from build123d import *
from OCP.BRepFilletAPI import BRepFilletAPI_MakeChamfer

# Parameters (mm, degrees)
SKETCH2_R           = 31
SKETCH2_R_2         = 25
SKETCH2_R_3         = 4
SKETCH2_R_4         = 3
SKETCH2_R_5         = 3.333333333
BOSS_EXTRUDE1_DEPTH = 10
BOSS_EXTRUDE2_START = 50
SKETCH2_3_R         = 31
SKETCH2_3_R_2       = 25
BOSS_EXTRUDE2_DEPTH = 50
FILLET1_R           = 6
SKETCH3_R           = 7
CUT_EXTRUDE1_DEPTH  = 3
BOSS_EXTRUDE3_DEPTH = 6
CIRPATTERN1_COUNT   = 6
BOSS_EXTRUDE4_START = 44
SKETCH6_R           = 70
SKETCH6_R_2         = 55
BOSS_EXTRUDE4_DEPTH = 6
CHAMFER1_SIZE       = 12.228610788
CHAMFER1_SIZE_2     = 24
CUT_EXTRUDE2_DEPTH  = 6
CIRPATTERN2_COUNT   = 12


with BuildPart() as part:
    # Sketch2 → Boss-Extrude1 (new body)
    # profile 1 of 2: a face of its own
    with BuildSketch(Plane(origin=(0, 0, 0), x_dir=(1, 0, 0), z_dir=(0, 1, 0))):
        with Locations(Location((0, 0, 0), (0, 0, 270))):
            Circle(SKETCH2_R)
        Circle(SKETCH2_R_2, mode=Mode.SUBTRACT)
    # profile 2 of 2: a face of its own
    with BuildSketch(Plane(origin=(0, 0, 0), x_dir=(1, 0, 0), z_dir=(0, 1, 0))):
        Circle(SKETCH2_R_2)
        with Locations(Location((0, 0, 0), (0, 0, 270))):
            Circle(SKETCH2_R_3, mode=Mode.SUBTRACT)
        with Locations(Location((-16, 0, 0), (0, 0, 270))):
            Circle(SKETCH2_R_4, mode=Mode.SUBTRACT)
        with Locations(Location((16, 0, 0), (0, 0, 270))):
            Circle(SKETCH2_R_5, mode=Mode.SUBTRACT)
    extrude(amount=-BOSS_EXTRUDE1_DEPTH)

    # Sketch2<3> → Boss-Extrude2 (add)
    with BuildSketch(Plane(origin=(0, 0, 0), x_dir=(1, 0, 0), z_dir=(0, 1, 0)).offset(BOSS_EXTRUDE2_START)):
        with Locations(Location((0, 0, 0), (0, 0, 270))):
            Circle(SKETCH2_3_R)
        with Locations(Location((0, 0, 0), (0, 0, 270))):
            Circle(SKETCH2_3_R_2, mode=Mode.SUBTRACT)
    extrude(amount=-BOSS_EXTRUDE2_DEPTH)

    # Fillet1
    fillet1_edges = [part.edges().sort_by_distance(p)[0] for p in [
        (0, -10, -31),
    ]]
    fillet(fillet1_edges, radius=FILLET1_R)

    # Sketch3 → Cut-Extrude1 (cut)
    with BuildSketch(Plane.XZ.offset(10)):
        with Locations(Location((16, 0, 0), (0, 0, 270))):
            Circle(SKETCH3_R)
        with Locations(Location((-16, 0, 0), (0, 0, 270))):
            Circle(SKETCH3_R)
    extrude(amount=-CUT_EXTRUDE1_DEPTH, mode=Mode.SUBTRACT)

    # Sketch4 → Boss-Extrude3 (add)
    with BuildSketch(Plane(origin=(0, 50, 0), x_dir=(1, 0, 0), z_dir=(0, 1, 0))):
        with BuildLine():
            ThreePointArc((0, 31), (1.500563555, 30.963661105), (2.997609122, 30.854729614))
            Line((2.997609122, 30.854729614), (2.997609122, 54.918251425))
            ThreePointArc((2.997609122, 54.918251425), (1.499361804, 54.979559058), (0, 55))
            Line((0, 55), (0, 31))
        make_face()
        with BuildLine():
            ThreePointArc((-2.997609122, 30.854729614), (-1.500563555, 30.963661105), (0, 31))
            Line((0, 31), (0, 55))
            ThreePointArc((0, 55), (-1.499361804, 54.979559058), (-2.997609122, 54.918251425))
            Line((-2.997609122, 54.918251425), (-2.997609122, 30.854729614))
        make_face()
    boss_extrude3 = extrude(amount=-BOSS_EXTRUDE3_DEPTH)

    # CirPattern1: Boss-Extrude3 ×6 about axis
    cirpattern1_axis = Axis((0, 0, 0), (0, 1, 0))
    for i in range(1, CIRPATTERN1_COUNT):
        add(boss_extrude3.rotate(cirpattern1_axis, i * 360 / CIRPATTERN1_COUNT))

    # Sketch6 → Boss-Extrude4 (add)
    with BuildSketch(Plane(origin=(0, 0, 0), x_dir=(1, 0, 0), z_dir=(0, 1, 0)).offset(BOSS_EXTRUDE4_START)):
        with Locations(Location((0, 0, 0), (0, 0, 270))):
            Circle(SKETCH6_R)
        Circle(SKETCH6_R_2, mode=Mode.SUBTRACT)
    extrude(amount=BOSS_EXTRUDE4_DEPTH)

    # Chamfer1
    chamfer1_edges_1 = [part.edges().sort_by_distance(p)[0] for p in [
        (0, 44, -31),
    ]]
    chamfer1_side_1 = [part.faces().sort_by_distance(p)[0] for p in [
        (0, 43.755427784, -31),
    ]]
    chamfer1_edges_2 = [part.edges().sort_by_distance(p)[0] for p in [
        (-26.846787517, 44, 15.5),
    ]]
    chamfer1_side_2 = [part.faces().sort_by_distance(p)[0] for p in [
        (-26.846787517, 43.755427784, 15.5),
    ]]
    chamfer1_edges_3 = [part.edges().sort_by_distance(p)[0] for p in [
        (-26.846787517, 44, -15.5),
    ]]
    chamfer1_side_3 = [part.faces().sort_by_distance(p)[0] for p in [
        (-26.846787517, 43.755427784, -15.5),
    ]]
    chamfer1_edges_4 = [part.edges().sort_by_distance(p)[0] for p in [
        (26.846787517, 44, -15.5),
    ]]
    chamfer1_side_4 = [part.faces().sort_by_distance(p)[0] for p in [
        (26.846787517, 43.755427784, -15.5),
    ]]
    chamfer1_edges_5 = [part.edges().sort_by_distance(p)[0] for p in [
        (26.846787517, 44, 15.5),
    ]]
    chamfer1_side_5 = [part.faces().sort_by_distance(p)[0] for p in [
        (26.846787517, 43.755427784, 15.5),
    ]]
    chamfer1_edges_6 = [part.edges().sort_by_distance(p)[0] for p in [
        (1.500563555, 44, 30.963661105),
    ]]
    chamfer1_side_6 = [part.faces().sort_by_distance(p)[0] for p in [
        (1.500563555, 43.755427784, 30.963661105),
    ]]
    chamfer1 = BRepFilletAPI_MakeChamfer(part.part.solid().wrapped)
    for e in chamfer1_edges_1:
        chamfer1.Add(CHAMFER1_SIZE - 0.0001, CHAMFER1_SIZE_2 - 0.0001, e.wrapped, chamfer1_side_1[0].wrapped)
    for e in chamfer1_edges_2:
        chamfer1.Add(CHAMFER1_SIZE - 0.0001, CHAMFER1_SIZE_2 - 0.0001, e.wrapped, chamfer1_side_2[0].wrapped)
    for e in chamfer1_edges_3:
        chamfer1.Add(CHAMFER1_SIZE - 0.0001, CHAMFER1_SIZE_2 - 0.0001, e.wrapped, chamfer1_side_3[0].wrapped)
    for e in chamfer1_edges_4:
        chamfer1.Add(CHAMFER1_SIZE - 0.0001, CHAMFER1_SIZE_2 - 0.0001, e.wrapped, chamfer1_side_4[0].wrapped)
    for e in chamfer1_edges_5:
        chamfer1.Add(CHAMFER1_SIZE - 0.0001, CHAMFER1_SIZE_2 - 0.0001, e.wrapped, chamfer1_side_5[0].wrapped)
    for e in chamfer1_edges_6:
        chamfer1.Add(CHAMFER1_SIZE - 0.0001, CHAMFER1_SIZE_2 - 0.0001, e.wrapped, chamfer1_side_6[0].wrapped)
    add(Compound.cast(chamfer1.Shape()), mode=Mode.REPLACE)  # a hair under: the kernel refuses the full size

    # Sketch7 → Cut-Extrude2 (cut)
    with BuildSketch(Plane(origin=(0, 50, 0), x_dir=(1, 0, 0), z_dir=(0, 1, 0))):
        with BuildLine():
            ThreePointArc((0, -60.5), (-2, -62.5), (0, -64.5))
            Line((0, -64.5), (0, -60.5))
        make_face()
        with BuildLine():
            Line((0, -60.5), (0, -64.5))
            ThreePointArc((0, -64.5), (1.414213562, -63.914213562), (2, -62.5))
            ThreePointArc((2, -62.5), (1.414213562, -61.085786438), (0, -60.5))
        make_face()
    cut_extrude2 = extrude(amount=-CUT_EXTRUDE2_DEPTH, mode=Mode.SUBTRACT)

    # CirPattern2: Cut-Extrude2 ×12 about axis
    cirpattern2_axis = Axis((0, 0, 0), (0, 1, 0))
    for i in range(1, CIRPATTERN2_COUNT):
        add(cut_extrude2.rotate(cirpattern2_axis, i * 360 / CIRPATTERN2_COUNT), mode=Mode.SUBTRACT)


solid = part.part
CAD build for the part. Positions are in the model's coordinates, mm. A direction names the side the tool comes from. Round coordinates to 2 decimals unless told otherwise and drop trailing zeros. Loops run counter-clockwise (first coordinate to the right, second up) from the corner with the lowest first, then second, coordinate; pieces in that order, holes last. Notation, with made-up numbers: (43.5, -16.75) - (53.5, -16.75) arc R12 cw to (53.5, -1.75) - close; hole circle Ø9 at (-23, 74.5). An arc over 180 degrees is marked (long way). Put each result on its own line as item: value.
1. Slice it at B-B on x = 43.5. Give the number of separate pieces and of enclosed holes in the cut face, and give its area (3 significant figures).
Geometry check:
separate pieces: 4
enclosed holes: 0
area: 371 mm²
2. Pin check, flat tips, straight feed: P1, Ø8, axis at x = -16, z = 0, coming from the +Y side; P2, Ø7, axis at x = -18, z = -2, coming from the -Y side; P3, Ø4, axis at x = 11, y = 23, coming from the -Z side; P4, Ø5.5, axis at x = 16, z = 0, coming from the -Y side. Stop position of each tip, or through.
Geometry check:
P1: y = 0
P2: y = -7
P3: z = -29.66
P4: through
3. 3-axis set-ups, long thin cutter, end or side, ignore diameter. For faces 5 (the flat face through (-30, 50, -1)), 6 (the flat face through (-2.998, 43, -40)), 7 (the cylindrical face through (-22.834, -8.521, 1.517)), 8 (the cylindrical face through (7.509, 25.35, 23.846)): which of +Z, -Z, +X, -X, +Y, -Y reach the whole face in a straight line?
Geometry check:
face 5: +Z, -Z, +X, -X, +Y
face 6: +Y, -Y
face 7: -Y
face 8: +Y
4. Two-plate mould, pull along Z, no slides. Class faces 1 (the flat face through (2.998, 43, 40)), 2 (the flat face through (5, -10, 0)), 3 (the cylindrical face through (-42.594, 46.958, -55.55)), 4 (the flat face through (33.18, 43.04, 22.62)): released by +Z, released by -Z, zero draft, split by the parting line, or undercut.
Geometry check:
face 1: undercut
face 2: zero draft
face 3: split by the parting line
face 4: undercut
5. Wall check: line 1 (X direction, y = -3.75, z = 0); line 2 (X direction, y = 38.5, z = -20); line 3 (Y direction, x = -53, z = -19). Give the ranges that are in metal, low to high.
Geometry check:
line 1: -31 to -19, -13 to -4, 4 to 12.67, 19.33 to 31
line 2: -39.42 to -28.65, -23.69 to -15, 15 to 23.69, 28.65 to 39.42
line 3: 44 to 50
6. Slice it at A-A on y = 29. List the corners of the cut face in (x, z).
Geometry check:
outline: circle Ø62 at (0, 0); hole circle Ø50 at (0, 0)
